Read the model definition and answer for the solid it produces. Units are mm, in the model's axes. Face numbers are marked on the shaded views. A direction names the side the tool comes from. Give positions to 0.01 mm unless a question says otherwise; leave off trailing zeros. Write each loop counter-clockwise with the first axis right and the second up, starting at its lowest first coordinate (ties: lowest second). Pieces come first, ordered by that corner, then holes. Notation, with made-up numbers: (-39.5, 11) -> (-3.5, 11) arc R24 ccw to (-3.5, 23) -> close; hole circle Ø9 at (85.25, 86.25). An arc over 180 degrees is marked (long way). Use a Markdown table: item, result.
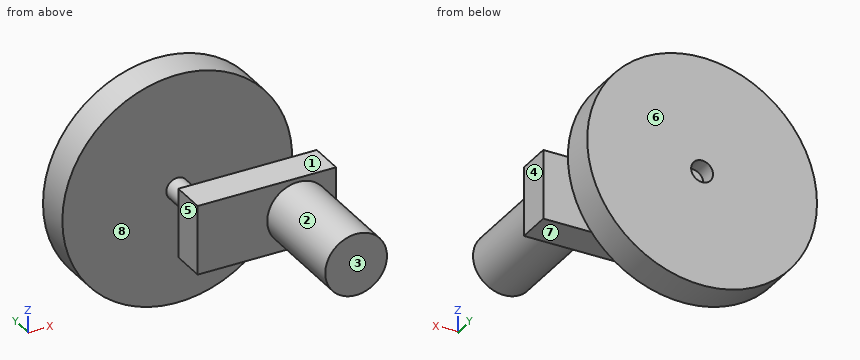
from build123d import *

# Parameters (mm, degrees)
F0_W     = 101.6
F0_H     = 50.8
F1_DEPTH = 25.4
F2_R     = 22.674477
F3_DEPTH = 76.2
F4_R     = 8.036326
F5_DEPTH = 50.8
F6_R     = 84.345052
F6_R_2   = 8.036326
F7_DEPTH = 12.7


with BuildPart() as f1:
    # F0 (on Front) → F1 (new body)
    with BuildSketch(Plane.XZ):
        with Locations((50.8, 25.4)):
            Rectangle(F0_W, F0_H)
    extrude(amount=F1_DEPTH)

    # F2 (on face) → F3 (join)
    with BuildSketch(Plane.XZ.offset(25.4)):
        with Locations((73.721826, 25.155274)):
            Circle(F2_R)
    extrude(amount=F3_DEPTH)

    # F4 (on face) → F5 (join)
    with BuildSketch(Plane(origin=(0, 0, 0), x_dir=(-1, 0, 0), z_dir=(0, 1, 0))):
        with Locations((-20.490019, 25.804443)):
            Circle(F4_R)
    extrude(amount=F5_DEPTH)

    # F6 (on face) → F7 (join, symmetric)
    with BuildSketch(Plane(origin=(0, 50.8, 0), x_dir=(-1, 0, 0), z_dir=(0, 1, 0))):
        with Locations((-20.490019, 25.804443)):
            Circle(F6_R)
        with Locations((-20.490019, 25.804443)):
            Circle(F6_R_2, mode=Mode.SUBTRACT)
    extrude(amount=F7_DEPTH, both=True)


solid = f1.part
Item 1: A tool of negligible diameter and unlimited length cuts with its end or side. For the marked faces 1, 2, 3, 4 and 5, from which of +Z, -Z, +X, -X, +Y, -Y can it reach the whole face along a straight path? Write none if from no direction.
Return value:
| item | result |
|---|---|
| face 1 | +Z, +X, -X, -Y |
| face 2 | -Y |
| face 3 | +Z, -Z, +X, -X, -Y |
| face 4 | +Z, -Z, +X, -Y |
| face 5 | +Z, -Z, -X, -Y |
Item 2: A cutting plane is placed at B-B (x = 32). Give the vertices of the cut face in (y, z).
Return value:
| item | result |
|---|---|
| outline | (-25.4, 0) -> (0, 0) -> (0, 50.8) -> (-25.4, 50.8) -> close; (38.1, -57.75) -> (63.5, -57.75) -> (63.5, 109.36) -> (38.1, 109.36) -> close |
Item 3: Straight lines are drawn through the part: line 1 along Y through (x, z) = (76.5, 15.5); line 2 along Y through (x, z) = (7, 35.5); line 3 along Y through (x, z) = (-12, 89). For each, find the intervals that lie inside material, in ascending order. Write a range as [from, to].
Return value:
| item | result |
|---|---|
| line 1 | [-101.6, 0], [38.1, 63.5] |
| line 2 | [-25.4, 0], [38.1, 63.5] |
| line 3 | [38.1, 63.5] |
Item 4: A cutting plane is placed at A-A (z = 40). Give the vertices of the cut face in (x, y).
Return value:
| item | result |
|---|---|
| outline | (-62.65, 38.1) -> (103.63, 38.1) -> (103.63, 63.5) -> (-62.65, 63.5) -> close; (0, -25.4) -> (56.58, -25.4) -> (56.58, -101.6) -> (90.86, -101.6) -> (90.86, -25.4) -> (101.6, -25.4) -> (101.6, 0) -> (0, 0) -> close |
Item 5: A cutting plane is placed at D-D (z = 10.5). Give the vertices of the cut face in (x, y).
Return value:
| item | result |
|---|---|
| outline | (-62.45, 38.1) -> (103.43, 38.1) -> (103.43, 63.5) -> (-62.45, 63.5) -> close; (0, -25.4) -> (56.42, -25.4) -> (56.42, -101.6) -> (91.02, -101.6) -> (91.02, -25.4) -> (101.6, -25.4) -> (101.6, 0) -> (0, 0) -> close |
Item 6: For a pull along Y with two mould halves and no side action, classify the marked faces 6, 7 and 8 as +Y half, -Y half, draft (parallel to the pull), parting line (faces both ways), or undercut.
Return value:
| item | result |
|---|---|
| face 6 | +Y half |
| face 7 | draft |
| face 8 | undercut |
Item 7: A cutting plane is placed at C-C (y = -10). Give the vertices of the cut face in (x, z), then the cut area to 3 significant figures.
Return value:
| item | result |
|---|---|
| outline | (0, 0) -> (101.6, 0) -> (101.6, 50.8) -> (0, 50.8) -> close |
| area | 5,160 mm^2 |
Item 8: Each of these flat-tipped pins is pushed along its axis until it touches: P1, Ø5, axis at x = 21.5, z = 23.5, coming from the +Y side; P2, Ø7.5, axis at x = 71, y = -8.5, coming from the -Z side; P3, Ø18.5, axis at x = 20.49, z = 25.8, coming from the -Y side. Where does it stop, or does it pass through?
Return value:
| item | result |
|---|---|
| P1 | y = 50.8 |
| P2 | z = 0 |
| P3 | y = -25.4 |
